from build123d import *

# Parameters (mm, degrees)
SKETCH3_R          = 0.75
SKETCH3_R_2        = 0.5
CUT_EXTRUDE1_DEPTH = 6
SKETCH3_3_R        = 1.5
CUT_EXTRUDE2_DEPTH = 2


with BuildPart() as part:
    # Sketch1 → Revolve1 (revolve)
    with BuildSketch(Plane(origin=(0, 0, 0), x_dir=(0, 0, -1), z_dir=(1, 0, 0))):
        Polygon((0, 0), (4, 0), (0, 6), align=None)
    revolve(axis=Axis((0, -11.26056338, 0), (0, 1, 0)))

    # Sketch3 → Cut-Extrude1 (cut)
    with BuildSketch(Plane.XZ):
        with Locations(Location((-2.5, 0, 0), (0, 0, 270))):
            Circle(SKETCH3_R)
        with Locations(Location((0, -2.5, 0), (0, 0, 270))):
            Circle(SKETCH3_R)
        with Locations(Location((2.5, 0, 0), (0, 0, 270))):
            Circle(SKETCH3_R)
        with Locations(Location((0, 0, 0), (0, 0, 270))):
            Circle(SKETCH3_R_2)
        with Locations(Location((0, 2.5, 0), (0, 0, 270))):
            Circle(SKETCH3_R)
    extrude(amount=-CUT_EXTRUDE1_DEPTH, mode=Mode.SUBTRACT)

    # Sketch3_3 → Cut-Extrude2 (cut)
    with BuildSketch(Plane.XZ):
        with Locations(Location((0, 0, 0), (0, 0, 270))):
            Circle(SKETCH3_3_R)
    extrude(amount=-CUT_EXTRUDE2_DEPTH, mode=Mode.SUBTRACT)


solid = part.part
Here's how the part is built. I have some questions about the finished solid (model axes, mm). A direction names the side the tool comes from. Coordinates: 2 decimals unless noted, no trailing zeros. Loops run counter-clockwise (first coordinate to the right, second up) from the corner with the lowest first, then second, coordinate; pieces in that order, holes last. Notation, with made-up numbers: (-36.75, 3.25) -> (15.25, 3.25) arc R21 cw to (15.25, 34.25) -> close; hole circle Ø4 at (9.25, 70). An arc over 180 degrees is marked (long way). Use one line per item in the form item = value. Start each with the question number.
(1) If we section it at C-C (y = 2.5): Please give me the cut outline in (x, z).
(2) If we section it at D-D (y = 4.6): Please give me the cut outline in (x, z).
(3) Will these pins go through, and if not, where does the flat tip stop? pin 1 (1.4 mm diameter, centred on x = -2.5, z = 0, fed in from -Y); pin 2 (2 mm diameter, centred on x = 2.5, z = 0, fed in from +Y); pin 3 (1 mm diameter, centred on y = 4, z = -0.5, fed in from +X); pin 4 (0.9 mm diameter, centred on x = -0.5, z = -0.5, fed in from -Y).
(4) If we section it at A-A (x = 0): Please give me the cut outline in (y, z) (3 decimals), then the cut area to 4 significant figures.
(5) Please list where these lines run through material, in increasing order: line 1 along X through (y, z) = (0.6, -0.5); line 2 along Z through (x, y) = (-1.25, 1.5); line 3 along Z through (x, y) = (2.5, 1.2).
(6) On a 3-axis mill with a long thin cutter (end or side, diameter ignored), from which of +Z, -Z, +X, -X, +Y, -Y can I reach the whole of each face in a straight line? I mean faces 1 (the face through (1.768, 1.289, 0.163)), 2 (the face through (0.45, 0.99, -1.43)). Say none if no direction works.
(7) We'd pull the mould along X, two halves only. Please class faces 3 (the face through (1, 0, 2)), 4 (the face through (0.55, 3.83, -1.34)), 5 (the face through (-0.488, 3.602, 0.108)): pulls with the +X half, pulls with the -X half, needs draft (parallel to the pull), parting line crosses it, or undercut.
(8) If we section it at B-B (z = 0): Please give me the cut outline in (x, y) (3 decimals), then the cut area to 4 significant figures.
Verdict:
q1.outline = (-2.23, -0.7) arc R2.33 ccw to (-0.7, -2.23) arc R0.75 cw to (0.7, -2.23) arc R2.33 ccw to (2.23, -0.7) arc R0.75 cw to (2.23, 0.7) arc R2.33 ccw to (0.7, 2.23) arc R0.75 cw to (-0.7, 2.23) arc R2.33 ccw to (-2.23, 0.7) arc R0.75 cw to start; hole circle Ø1 at (0, 0)
q2.outline = circle Ø1.87 at (0, 0); hole circle Ø1 at (0, 0)
q3.pin_1 = through
q3.pin_2 = 3.75
q3.pin_3 = 1.61
q3.pin_4 = 2
q4.outline = (0, -4) -> (1.125, -3.25) -> (0, -3.25) -> close; (0, -1.75) -> (3.375, -1.75) -> (5.25, -0.5) -> (2, -0.5) -> (2, -1.5) -> (0, -1.5) -> close; (0, 1.5) -> (2, 1.5) -> (2, 0.5) -> (5.25, 0.5) -> (3.375, 1.75) -> (0, 1.75) -> close; (0, 3.25) -> (1.125, 3.25) -> (0, 4) -> close
q4.area = 7.625 mm²
q5.line_1 = -3.57 to -3.06, -1.94 to -1.41, 1.41 to 1.94, 3.06 to 3.57
q5.line_2 = -2.73 to -0.83, 0.83 to 2.73
q5.line_3 = -2 to -0.75, 0.75 to 2
q6.face_1 = +Y, -Y
q6.face_2 = -Y
q7.face_3 = needs draft
q7.face_4 = parting line crosses it
q7.face_5 = undercut
q8.outline = (-4, 0) -> (-3.25, 0) -> (-3.25, 1.125) -> close; (-1.75, 0) -> (-1.5, 0) -> (-1.5, 2) -> (-0.5, 2) -> (-0.5, 5.25) -> (-1.75, 3.375) -> close; (0.5, 2) -> (1.5, 2) -> (1.5, 0) -> (1.75, 0) -> (1.75, 3.375) -> (0.5, 5.25) -> close; (3.25, 0) -> (4, 0) -> (3.25, 1.125) -> close
q8.area = 7.625 mm²
